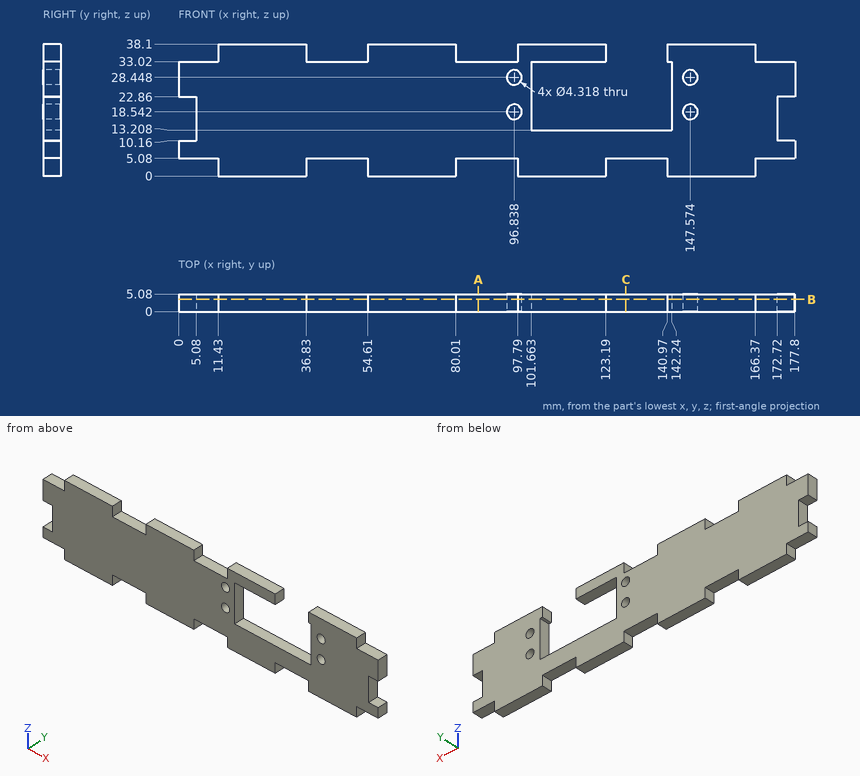
Can you work these out from the drawing? Everything is in mm from the part's minimum corner. Round coordinates to 2 decimals unless told otherwise and drop trailing zeros. Write each loop counter-clockwise with the first axis right and the second up, starting at its lowest first coordinate (ties: lowest second). Pieces come first, ordered by that corner, then holes. Notation, with made-up numbers: (-26, 12.25) - (19, 12.25) arc R13 ccw to (19, 16.25) - close; hole circle Ø5 at (70.25, 11). An arc over 180 degrees is marked (long way). Use a Markdown table: item, result.
Q1. I want a section at A-A (x = 86.5). List the corners of the cut face in (y, z) for me, plus the area to 3 significant figures.
Output values:
| item | result |
|---|---|
| outline | (0, 5.08) - (5.08, 5.08) - (5.08, 33.02) - (0, 33.02) - close |
| area | 142 mm2 |
Q2. Please list where these lines run through material, in increasing order: L1, parallel to X at y = 1, z = 28.5 (1 decimal); L2, parallel to X at y = 1.3, z = 4; L3, parallel to Z at x = 110, y = 2.9.
Output values:
| item | result |
|---|---|
| L1 | 0 to 94.7, 99 to 101.7, 142.2 to 145.4, 149.7 to 177.8 |
| L2 | 11.43 to 36.83, 54.61 to 80.01, 97.79 to 123.19, 140.97 to 166.37 |
| L3 | 0 to 13.21, 33.02 to 38.1 |
Q3. I want a section at B-B (y = 3.55). Count the separate pieces of the cut face and the enclosed holes in it, plus the area to 3 significant figures.
Output values:
| item | result |
|---|---|
| separate pieces | 1 |
| enclosed holes | 4 |
| area | 5,010 mm2 |
Q4. For pin 1 (1.5 mm diameter, centred on y = 3.5, z = 36.5, fed in from -X); pin 2 (1.5 mm diameter, centred on x = 170.5, y = 3, fed in from +Z); pin 3 (2.5 mm diameter, centred on y = 2, z = 2, fed in from +X); pin 4 (4 mm diameter, centred on x = 147.574, z = 28.448, fed in from +Y), each with a flat end and sliding along its axis, tell me the tip position at first contact or that it passes through.
Output values:
| item | result |
|---|---|
| pin 1 | x = 11.43 |
| pin 2 | z = 33.02 |
| pin 3 | x = 166.37 |
| pin 4 | through |
Q5. I want a section at C-C (x = 129). List the corners of the cut face in (y, z) for me, plus the area to 3 significant figures.
Output values:
| item | result |
|---|---|
| outline | (0, 5.08) - (5.08, 5.08) - (5.08, 13.21) - (0, 13.21) - close |
| area | 41.3 mm2 |
